from build123d import *

# Parameters (mm, degrees)
SKETCH1_R                                           = 1.55
BOSS_EXTRUDE1_DEPTH                                 = 27.8
SKETCH2_W                                           = 14
SKETCH2_H                                           = 5.2
CUT_EXTRUDE1_DEPTH                                  = 6.8
CBORE_FOR_M3_HEX_SOCKET_HEAD_CAP_SCREW1_D           = 3.6
CBORE_FOR_M3_HEX_SOCKET_HEAD_CAP_SCREW1_CBORE_D     = 6.5
CBORE_FOR_M3_HEX_SOCKET_HEAD_CAP_SCREW1_CBORE_DEPTH = 3.4
SKETCH6_W                                           = 27.8
SKETCH6_H                                           = 13
CUT_EXTRUDE2_DEPTH                                  = 0.7
FILLET1_R                                           = 2
FILLET2_R                                           = 1.4


with BuildPart() as part:
    # Sketch1 → Boss-Extrude1 (new body)
    with BuildSketch(Plane(origin=(0, 0, 0), x_dir=(0, 0, -1), z_dir=(1, 0, 0))):
        Polygon((0, 0), (13, 0), (13, 13.5), (5.2, 13.5), (5.2, 5.8), (0, 5.8), align=None)
        with Locations((10, 10.75)):
            Circle(SKETCH1_R, mode=Mode.SUBTRACT)
    extrude(amount=BOSS_EXTRUDE1_DEPTH)

    # Sketch2 → Cut-Extrude1 (cut, through all)
    with BuildSketch(Plane(origin=(0, 5.8, 0), x_dir=(1, 0, 0), z_dir=(0, 1, 0))):
        with Locations((13.9, 2.6)):
            Rectangle(SKETCH2_W, SKETCH2_H)
    extrude(amount=-CUT_EXTRUDE1_DEPTH, mode=Mode.SUBTRACT)

    # CBORE for M3 Hex Socket Head Cap Screw1 (through all)
    with Locations(Plane(origin=(0, 0, -13), x_dir=(-1, 0, 0), z_dir=(0, 0, -1))):
        with Locations((-13.9, 3)):
            CounterBoreHole(CBORE_FOR_M3_HEX_SOCKET_HEAD_CAP_SCREW1_D / 2, CBORE_FOR_M3_HEX_SOCKET_HEAD_CAP_SCREW1_CBORE_D / 2, CBORE_FOR_M3_HEX_SOCKET_HEAD_CAP_SCREW1_CBORE_DEPTH)

    # Sketch6 → Cut-Extrude2 (cut)
    with BuildSketch(Plane.XZ):
        with Locations((13.9, -6.5)):
            Rectangle(SKETCH6_W, SKETCH6_H)
    extrude(amount=-CUT_EXTRUDE2_DEPTH, mode=Mode.SUBTRACT)

    # Fillet1
    fillet1_edges = [part.edges().sort_by_distance(p)[0] for p in [
        (27.8, 5.8, -2.6),
        (0, 0.7, -6.5),
        (27.8, 0.7, -6.5),
        (0, 5.8, -2.6),
    ]]
    fillet(fillet1_edges, radius=FILLET1_R)

    # Fillet2
    fillet2_edges = [part.edges().sort_by_distance(p)[0] for p in [
        (6.80190375, 0.7, -13),
        (0, 8.1, -13),
        (0.585786438, 1.285786438, -13),
        (27.214213562, 1.285786438, -13),
        (13.9, 13.5, -13),
        (13.9, 6.25, -13),
        (20.99809625, 0.7, -13),
        (27.8, 8.1, -13),
    ]]
    fillet(fillet2_edges, radius=FILLET2_R)


solid = part.part
CAD build for the part. Positions are in the model's coordinates, mm. A direction names the side the tool comes from. Give positions to 0.01 mm unless a question says otherwise; leave off trailing zeros. Write each loop counter-clockwise with the first axis right and the second up, starting at its lowest first coordinate (ties: lowest second). Pieces come first, ordered by that corner, then holes. Notation, with made-up numbers: M 68.5,-14.5 L 111.5,-14.5 A27 cw 111.5,22.5 Z; hole C -27,-23 d10. An arc over 180 degrees is marked long. Put each result on its own line as item: value. Start each with the question number.
(1) Band-saw the part on C-C, the plane z = -5.75. Write the cut outline in (x, y), and give its area (3 significant figures).
(2) Probe L1, parallel to X at y = 3, z = -10.2; L2, parallel to Z at x = 20.75, y = 3.75; L3, parallel to Y at x = 6, z = -4. List the from-to ranges inside material, lowest first.
(3) Band-saw the part on D-D, the plane x = 7.75. Write the cut outline in (y, z).
(4) Band-saw the part on A-A, the plane z = -10. Write the cut outline in (x, y).
(5) Mould opens along Y. For faces 5 (the face through (6.9, 3, -3)), 6 (the face through (27.2, 1.27, -5.72)), 7 (the face through (23, 5.8, -3)), 8 (the face through (12.1, 3.08, -7.37)) say: +Y half, -Y half, draft (parallel to the pull), parting line (faces both ways), or undercut.
(6) Flat gauge pins, fed straight in: pin 1 Ø4.5 at (x, y) = (13, 3) entering from -Z; pin 2 Ø3 at (x, y) = (16, 11) entering from +Z; pin 3 Ø1.5 at (x, z) = (22.5, -3) entering from +Y. Where does each tip first touch, or does it go through?
(7) Which spindle directions (+Z, -Z, +X, -X, +Y, -Y) get a long thin tool onto all of the face, cutting with end or side? Do faces 1 (the face through (14.09, 13.1, -12.58)), 2 (the face through (27.23, 5.2, -2.56)), 3 (the face through (0.57, 5.2, -2.56)), 4 (the face through (15, 5, -9.6)). Say none if no direction does.
(8) Band-saw the part on B-B, the plane y = 10.75. Write the cut outline in (x, z), and give its area (3 significant figures).
Response values:
1. outline: M 0,2.7 A2 ccw 2,0.7 L 25.8,0.7 A2 ccw 27.8,2.7 L 27.8,13.5 L 0,13.5 Z; hole C 13.9,3 d3.6
1. area: 344 mm2
2. L1: x = 0 to 10.65, 17.15 to 27.8
2. L2: z = -13 to -5.2
2. L3: y = 0.7 to 5.8
3. outline: M 0.7,-11.6 A1.4 ccw 2.1,-13 L 12.1,-13 A1.4 ccw 13.5,-11.6 L 13.5,-5.2 L 0.7,-5.2 Z; hole C 10.75,-10 d3.1
4. outline: M 0,2.7 A2 ccw 2,0.7 L 11.6,0.7 A3.25 cw long 16.2,0.7 L 25.8,0.7 A2 ccw 27.8,2.7 L 27.8,9.2 L 0,9.2 Z; M 0,12.3 L 27.8,12.3 L 27.8,13.5 L 0,13.5 Z
5. face 5: draft
5. face 6: -Y half
5. face 7: +Y half
5. face 8: undercut
6. pin 1: stops at z = -9.6
6. pin 2: stops at z = -5.2
6. pin 3: stops at y = 5.8
7. face 1: -Z, +X, -X, +Y
7. face 2: +Z, +X, +Y
7. face 3: +Z, -X, +Y
7. face 4: -Z
8. outline: M 0,-11.6 A1.4 ccw 1.4,-13 L 26.4,-13 A1.4 ccw 27.8,-11.6 L 27.8,-11.55 L 0,-11.55 Z; M 0,-8.45 L 27.8,-8.45 L 27.8,-5.2 L 0,-5.2 Z
8. area: 130 mm2
